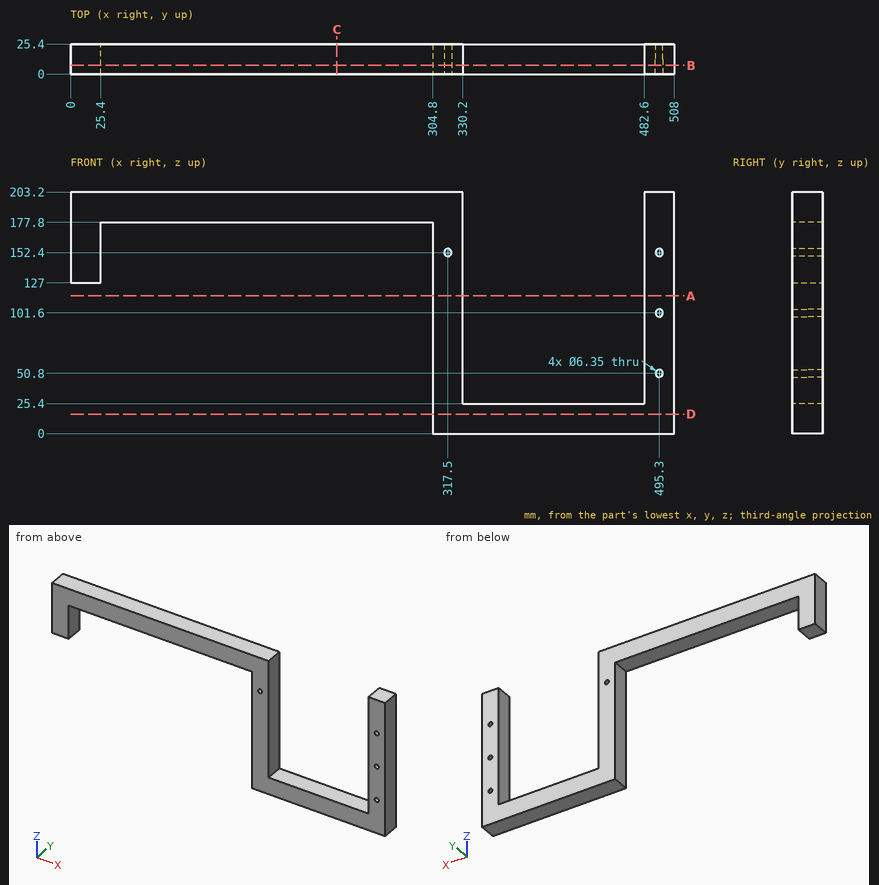
Source: three-view drawing plus pictorial views. Frame: mm from the lowest corner of the part. Give positions to 0.01 mm unless a question says otherwise; leave off trailing zeros. Write each loop counter-clockwise with the first axis right and the second up, starting at its lowest first coordinate (ties: lowest second). Pieces come first, ordered by that corner, then holes.
(1) Ray query, line 1 (X direction, y = 6, z = 101.6) (3 decimals); line 2 (X direction, y = 15.75, z = 93); line 3 (X direction, y = 23.25, z = 169.5). Return the intervals inside material, ascending.
(2) Cut plane B-B, the plane y = 7.5. Return loops of the section in (x, z) (3 decimals), then the cut area to 3 significant figures.
(3) Cut plane D-D, the plane z = 16.5. Return loops of the section in (x, y).
(4) Cut plane A-A, the plane z = 116. Return loops of the section in (x, y).
(5) Cut plane C-C, the plane x = 224. Return loops of the section in (y, z), then the cut area to 3 significant figures.
(6) First-contact query: P1, Ø7.5, axis at x = 495.3, z = 152.4, coming from the +Y side; P2, Ø10, axis at y = 10, z = 90, coming from the -X side; P3, Ø4, axis at x = 495.3, z = 152.4, coming from the +Y side; P4, Ø7.5, axis at x = 9, y = 10, coming from the -Z side. Flat tips, straight axial feed; report the tip coordinate or a pass-through.
Values follow:
1. line 1: x = 304.8 to 330.2, 482.6 to 492.125, 498.475 to 508
1. line 2: x = 304.8 to 330.2, 482.6 to 508
1. line 3: x = 0 to 25.4, 304.8 to 330.2, 482.6 to 508
2. outline: (0, 127) - (25.4, 127) - (25.4, 177.8) - (304.8, 177.8) - (304.8, 0) - (508, 0) - (508, 203.2) - (482.6, 203.2) - (482.6, 25.4) - (330.2, 25.4) - (330.2, 203.2) - (0, 203.2) - close; hole circle Ø6.35 at (317.5, 152.4); hole circle Ø6.35 at (495.3, 50.8); hole circle Ø6.35 at (495.3, 101.6); hole circle Ø6.35 at (495.3, 152.4)
2. area: 23,100 mm2
3. outline: (304.8, 0) - (508, 0) - (508, 25.4) - (304.8, 25.4) - close
4. outline: (304.8, 0) - (330.2, 0) - (330.2, 25.4) - (304.8, 25.4) - close; (482.6, 0) - (508, 0) - (508, 25.4) - (482.6, 25.4) - close
5. outline: (0, 177.8) - (25.4, 177.8) - (25.4, 203.2) - (0, 203.2) - close
5. area: 645 mm2
6. P1: stops at y = 25.4
6. P2: stops at x = 304.8
6. P3: passes through
6. P4: stops at z = 127
